Geometry: final body of the model. Coordinates: model frame, mm. Coordinates: 2 decimals unless noted, no trailing zeros. Loops run counter-clockwise (first coordinate to the right, second up) from the corner with the lowest first, then second, coordinate; pieces in that order, holes last. Notation, with made-up numbers: (76, 63.25) -> (107, 63.25) arc R18 cw to (107, 69.25) -> close; hole circle Ø4 at (29, 14). An arc over 180 degrees is marked (long way). One line per item, written item: value. Start each with the question number.
Item 1: Ray query, probe 1 along Z at (x, y) = (25, -3); probe 2 along X at (y, z) = (-3.65, -62) (3 decimals). Return the intervals inside material, ascending. Write a range as from..to.
Item 2: Section query A-A on x = 2.5. Return loops of the section in (y, z).
Item 3: Section query B-B on z = -28.5. Return loops of the section in (x, y) (3 decimals), then the cut area to 3 significant figures.
Item 4: Contact query for flat-ended pins moving along their axis: pin 1 Ø1 at (x, y) = (1.5, -3.5) entering from -Z; pin 2 Ø2.5 at (x, y) = (21, -2.5) entering from -Z. Output: stop coordinate, or through.
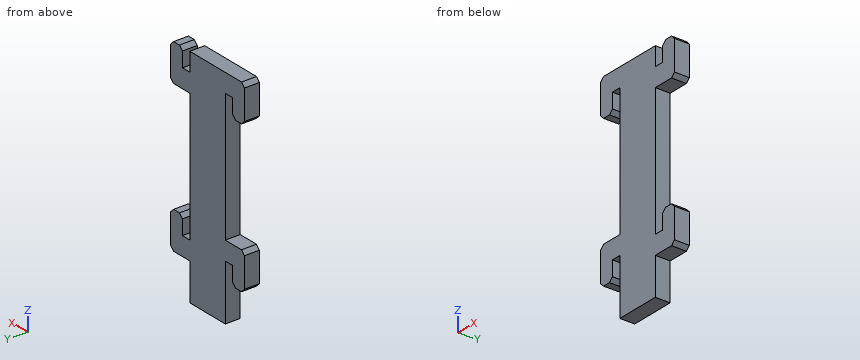
from build123d import *

# Parameters (mm, degrees)
F1_DEPTH = 5.08
F2_SIZE  = 1.27


with BuildPart() as f1:
    # F0 (on Front) → F1 (new body)
    with BuildSketch(Plane.XZ):
        Polygon((0, -6.35), (0, 0), (3.175, 0), (3.175, -44.45), (3.175, -50.8), (18.415, -50.8), (18.415, -6.35), (18.415, 0), (18.415, 6.35), (3.175, 6.35), (-5.08, 6.35), (-5.08, -6.35), align=None)
        Polygon((3.175, -50.8), (3.175, -44.45), (-5.08, -44.45), (-5.08, -57.15), (0, -57.15), (0, -50.8), (0.926509, -50.8), align=None)
        Polygon((18.415, -50.8), (3.175, -50.8), (3.175, -69.85), (18.415, -69.85), (18.415, -57.15), align=None)
        Polygon((21.59, -50.8), (18.415, -50.8), (18.415, -57.15), (26.67, -57.15), (26.67, -44.45), (21.59, -44.45), align=None)
        Polygon((18.415, 0), (18.415, -6.35), (26.67, -6.35), (26.67, 6.35), (21.59, 6.35), (21.59, 0), align=None)
    extrude(amount=F1_DEPTH)

    # F2
    f2_edges = [f1.edges().sort_by_distance(p)[0] for p in [
        (21.59, -2.54, 6.35),
        (26.67, -2.54, 6.35),
        (26.67, -2.54, -6.35),
        (0, -2.54, -6.35),
        (-5.08, -2.54, -6.35),
        (-5.08, -2.54, 6.35),
        (26.67, -2.54, -44.45),
        (21.59, -2.54, -44.45),
        (26.67, -2.54, -57.15),
        (-5.08, -2.54, -44.45),
        (-5.08, -2.54, -57.15),
        (0, -2.54, -57.15),
    ]]
    chamfer(f2_edges, length=F2_SIZE)


solid = f1.part
Reply:
1. probe 1: z = -57.15..-44.45, -6.35..6.35
1. probe 2: x = 3.175..18.415
2. outline: (-5.08, -50.8) -> (0, -50.8) -> (0, -44.45) -> (-5.08, -44.45) -> close; (-5.08, 0) -> (0, 0) -> (0, 6.35) -> (-5.08, 6.35) -> close
3. outline: (3.175, -5.08) -> (18.415, -5.08) -> (18.415, 0) -> (3.175, 0) -> close
3. area: 77.4 mm²
4. pin 1: stops at z = -50.8
4. pin 2: stops at z = -57.15
